Geometry check sheet. Reference: the model listing, model coordinates, mm. Give positions to 0.01 mm unless a question says otherwise; leave off trailing zeros. Write each loop counter-clockwise with the first axis right and the second up, starting at its lowest first coordinate (ties: lowest second). Pieces come first, ordered by that corner, then holes.
(1) Thickness scan on line 1 along Z through (x, y) = (-31.5, 1.6); line 2 along X through (y, z) = (1.5, 15); line 3 along X through (y, z) = (0.9, -33.5). Record the ranges inside material, lowest first.
(2) Cross-section at B-B (z = 25). Record the boundary of the cut face in (x, y), and give its area (3 significant figures).
(3) Cross-section at C-C (x = 42). Record the boundary of the cut face in (y, z).
(4) Cross-section at A-A (y = 1.3). Record the boundary of the cut face in (x, z).
Autodesk Inventor part; units mm, degrees
ref_plane "YZ Plane" through (0, 0, 0) normal (1, 0, 0) x (0, 1, 0)
ref_plane "XZ Plane" through (0, 0, 0) normal (0, 1, 0) x (-1, 0, 0)
ref_plane "XY Plane" through (0, 0, 0) normal (0, 0, 1) x (1, 0, 0)
sketch "Sketch1" plane through (0, 0, 0) normal (0, 1, 0) x (-1, 0, 0)
  line L0 (-29.1562, -50.5) -> (-58.3124, 0)
  line L1 (-58.3124, 0) -> (-29.1562, 50.5)
  line L2 (-29.1562, 50.5) -> (29.1562, 50.5)
  line L3 (29.1562, 50.5) -> (58.3124, 0)
  line L4 (58.3124, 0) -> (29.1562, -50.5)
  line L5 (29.1562, -50.5) -> (-29.1562, -50.5)
  point P0 (0, 0)
  point P1 (0, 0)
  dimension "d0" = 101
extrude "Extrusion1" add sketch "Sketch1" along normal blind 1.7
equation "\"d0\" = FlatDiameter"
equation "\"d1\" = Thickness"
equation "\"FlatDiameter\" = 101"
equation "\"Thickness\" = 1.7"
properties part number "Hex_Single" material "Paper"
Reply:
1. line 1: z = -46.44 to 46.44
1. line 2: x = -49.65 to 49.65
1. line 3: x = -38.97 to 38.97
2. outline: (-43.88, 0) - (43.88, 0) - (43.88, 1.7) - (-43.88, 1.7) - close
2. area: 149 mm2
3. outline: (0, -28.25) - (1.7, -28.25) - (1.7, 28.25) - (0, 28.25) - close
4. outline: (-58.31, 0) - (-29.16, -50.5) - (29.16, -50.5) - (58.31, 0) - (29.16, 50.5) - (-29.16, 50.5) - close
